Source: CAD feature listing. Evaluate the final solid. Frame: model axes, mm. Round coordinates to 2 decimals unless told otherwise and drop trailing zeros. Write each loop counter-clockwise with the first axis right and the second up, starting at its lowest first coordinate (ties: lowest second). Pieces come first, ordered by that corner, then holes. Notation, with made-up numbers: (32, 40) - (40, 40) arc R30 ccw to (40, 75) - close; hole circle Ø4 at (-6.75, 32.25). An arc over 180 degrees is marked (long way). Write item = value, one per line. Start each with the question number.
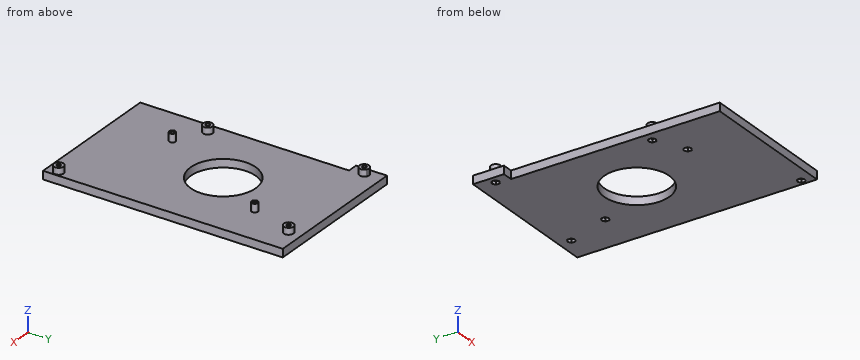
```python
from build123d import *

# Parameters (mm, degrees)
SKETCH1_R           = 20
SKETCH1_R_2         = 1.25
BOSS_EXTRUDE1_DEPTH = 5
BOSS_EXTRUDE2_START = 4
SKETCH1_3_R         = 1.25
SKETCH1_3_R_2       = 3
BOSS_EXTRUDE2_DEPTH = 4
BOSS_EXTRUDE3_START = 5
SKETCH1_5_R         = 1.9
SKETCH1_5_R_2       = 1.25
BOSS_EXTRUDE3_DEPTH = 5
CUT_EXTRUDE1_DEPTH  = 2
INTERSECT1_START    = -101.6
INTERSECT1_DEPTH    = 170


# Read off the part's stored shape, not the designer's step: Intersect1
with BuildPart() as part:
    # Sketch1 → Boss-Extrude1 (new body)
    with BuildSketch(Plane(origin=(0, 0, 0), x_dir=(0, 1, 0), z_dir=(0, 0, 1))):
        Polygon((-101.6, 25.4), (-101.6, -81.5), (215.9, -81.5), (215.9, 12.7), (196.85, 12.7), (196.85, 6.35), (-57.15, 6.35), (-57.15, 25.4), align=None)
        with Locations(Location((148.3, -36, 0), (0, 0, 270))):
            Circle(SKETCH1_R, mode=Mode.SUBTRACT)
        with Locations(Location((-92.5, 8, 0), (0, 0, 270))):
            Circle(SKETCH1_R_2, mode=Mode.SUBTRACT)
        with Locations(Location((205.3, 7.8, 0), (0, 0, 270))):
            Circle(SKETCH1_R_2, mode=Mode.SUBTRACT)
        with Locations(Location((-86.5, -73, 0), (0, 0, 270))):
            Circle(SKETCH1_R_2, mode=Mode.SUBTRACT)
        with Locations(Location((0, 0, 0), (0, 0, 270))):
            Circle(SKETCH1_R_2, mode=Mode.SUBTRACT)
        with Locations(Location((114.3, 0, 0), (0, 0, 270))):
            Circle(SKETCH1_R_2, mode=Mode.SUBTRACT)
        with Locations(Location((104.8, -18, 0), (0, 0, 270))):
            Circle(SKETCH1_R_2, mode=Mode.SUBTRACT)
        with Locations(Location((75.7, -78, 0), (0, 0, 270))):
            Circle(SKETCH1_R_2, mode=Mode.SUBTRACT)
        with Locations(Location((181.3, -56, 0), (0, 0, 270))):
            Circle(SKETCH1_R_2, mode=Mode.SUBTRACT)
        with Locations(Location((208.3, -65, 0), (0, 0, 270))):
            Circle(SKETCH1_R_2, mode=Mode.SUBTRACT)
    extrude(amount=-BOSS_EXTRUDE1_DEPTH)

    # Sketch1<3> → Boss-Extrude2 (add)
    # profile 1 of 9: a face of its own
    with BuildSketch(Plane(origin=(0, 0, 0), x_dir=(0, 1, 0), z_dir=(0, 0, 1)).offset(BOSS_EXTRUDE2_START)):
        with BuildLine():
            Line((-95.005493963, 6.35), (-89.994506037, 6.35))
            ThreePointArc((-89.994506037, 6.35), (-89.62628447, 7.13874565), (-89.5, 8))
            ThreePointArc((-89.5, 8), (-93.36125435, 10.87371553), (-95.005493963, 6.35))
        make_face()
        with Locations(Location((-92.5, 8, 0), (0, 0, 270))):
            Circle(SKETCH1_3_R, mode=Mode.SUBTRACT)
    # profile 2 of 9: a face of its own
    with BuildSketch(Plane(origin=(0, 0, 0), x_dir=(0, 1, 0), z_dir=(0, 0, 1)).offset(BOSS_EXTRUDE2_START)):
        with BuildLine():
            ThreePointArc((-95.005493963, 6.35), (-92.5, 5), (-89.994506037, 6.35))
            Line((-89.994506037, 6.35), (-95.005493963, 6.35))
        make_face()
    # profile 3 of 9: a face of its own
    with BuildSketch(Plane(origin=(0, 0, 0), x_dir=(0, 1, 0), z_dir=(0, 0, 1)).offset(BOSS_EXTRUDE2_START)):
        with Locations(Location((-86.5, -73, 0), (0, 0, 270))):
            Circle(SKETCH1_3_R_2)
        with Locations(Location((-86.5, -73, 0), (0, 0, 270))):
            Circle(SKETCH1_3_R, mode=Mode.SUBTRACT)
    # profile 4 of 9: a face of its own
    with BuildSketch(Plane(origin=(0, 0, 0), x_dir=(0, 1, 0), z_dir=(0, 0, 1)).offset(BOSS_EXTRUDE2_START)):
        with Locations(Location((0, 0, 0), (0, 0, 270))):
            Circle(SKETCH1_3_R_2)
        with Locations(Location((0, 0, 0), (0, 0, 270))):
            Circle(SKETCH1_3_R, mode=Mode.SUBTRACT)
    # profile 5 of 9: a face of its own
    with BuildSketch(Plane(origin=(0, 0, 0), x_dir=(0, 1, 0), z_dir=(0, 0, 1)).offset(BOSS_EXTRUDE2_START)):
        with Locations(Location((75.7, -78, 0), (0, 0, 270))):
            Circle(SKETCH1_3_R_2)
        with Locations(Location((75.7, -78, 0), (0, 0, 270))):
            Circle(SKETCH1_3_R, mode=Mode.SUBTRACT)
    # profile 6 of 9: a face of its own
    with BuildSketch(Plane(origin=(0, 0, 0), x_dir=(0, 1, 0), z_dir=(0, 0, 1)).offset(BOSS_EXTRUDE2_START)):
        with Locations(Location((114.3, 0, 0), (0, 0, 270))):
            Circle(SKETCH1_3_R_2)
        with Locations(Location((114.3, 0, 0), (0, 0, 270))):
            Circle(SKETCH1_3_R, mode=Mode.SUBTRACT)
    # profile 7 of 9: a face of its own
    with BuildSketch(Plane(origin=(0, 0, 0), x_dir=(0, 1, 0), z_dir=(0, 0, 1)).offset(BOSS_EXTRUDE2_START)):
        with Locations(Location((208.3, -65, 0), (0, 0, 270))):
            Circle(SKETCH1_3_R_2)
        with Locations(Location((208.3, -65, 0), (0, 0, 270))):
            Circle(SKETCH1_3_R, mode=Mode.SUBTRACT)
    # profile 8 of 9: a face of its own
    with BuildSketch(Plane(origin=(0, 0, 0), x_dir=(0, 1, 0), z_dir=(0, 0, 1)).offset(BOSS_EXTRUDE2_START)):
        with BuildLine():
            ThreePointArc((208.3, 7.8), (204.551310342, 10.705075523), (202.673690803, 6.35))
            Line((202.673690803, 6.35), (207.926309197, 6.35))
            ThreePointArc((207.926309197, 6.35), (208.205075523, 7.051310342), (208.3, 7.8))
        make_face()
        with Locations(Location((205.3, 7.8, 0), (0, 0, 270))):
            Circle(SKETCH1_3_R, mode=Mode.SUBTRACT)
    # profile 9 of 9: a face of its own
    with BuildSketch(Plane(origin=(0, 0, 0), x_dir=(0, 1, 0), z_dir=(0, 0, 1)).offset(BOSS_EXTRUDE2_START)):
        with BuildLine():
            Line((207.926309197, 6.35), (202.673690803, 6.35))
            ThreePointArc((202.673690803, 6.35), (205.3, 4.8), (207.926309197, 6.35))
        make_face()
    extrude(amount=-BOSS_EXTRUDE2_DEPTH)

    # Sketch1<5> → Boss-Extrude3 (add)
    # profile 1 of 2: a face of its own
    with BuildSketch(Plane(origin=(0, 0, 0), x_dir=(0, 1, 0), z_dir=(0, 0, 1)).offset(BOSS_EXTRUDE3_START)):
        with Locations(Location((104.8, -18, 0), (0, 0, 270))):
            Circle(SKETCH1_5_R)
        with Locations(Location((104.8, -18, 0), (0, 0, 270))):
            Circle(SKETCH1_5_R_2, mode=Mode.SUBTRACT)
    # profile 2 of 2: a face of its own
    with BuildSketch(Plane(origin=(0, 0, 0), x_dir=(0, 1, 0), z_dir=(0, 0, 1)).offset(BOSS_EXTRUDE3_START)):
        with Locations(Location((181.3, -56, 0), (0, 0, 270))):
            Circle(SKETCH1_5_R)
        with Locations(Location((181.3, -56, 0), (0, 0, 270))):
            Circle(SKETCH1_5_R_2, mode=Mode.SUBTRACT)
    extrude(amount=-BOSS_EXTRUDE3_DEPTH)

    # Sketch3 → Cut-Extrude1 (cut)
    with BuildSketch(Plane(origin=(0, 0, -5), x_dir=(1, 0, 0), z_dir=(0, 0, -1))):
        Polygon((78, -78.067136104), (80.05, -76.883568052), (80.05, -74.516431948), (78, -73.332863896), (75.95, -74.516431948), (75.95, -76.883568052), align=None)
        Polygon((65, -210.667136104), (67.05, -209.483568052), (67.05, -207.116431948), (65, -205.932863896), (62.95, -207.116431948), (62.95, -209.483568052), align=None)
        Polygon((56, -183.667136104), (58.05, -182.483568052), (58.05, -180.116431948), (56, -178.932863896), (53.95, -180.116431948), (53.95, -182.483568052), align=None)
        Polygon((-7.8, -207.667136104), (-5.75, -206.483568052), (-5.75, -204.116431948), (-7.8, -202.932863896), (-9.85, -204.116431948), (-9.85, -206.483568052), align=None)
        Polygon((0, -116.667136104), (2.05, -115.483568052), (2.05, -113.116431948), (0, -111.932863896), (-2.05, -113.116431948), (-2.05, -115.483568052), align=None)
        Polygon((18, -107.167136104), (20.05, -105.983568052), (20.05, -103.616431948), (18, -102.432863896), (15.95, -103.616431948), (15.95, -105.983568052), align=None)
        Polygon((0, -2.367136104), (2.05, -1.183568052), (2.05, 1.183568052), (0, 2.367136104), (-2.05, 1.183568052), (-2.05, -1.183568052), align=None)
        Polygon((-8, 90.132863896), (-5.95, 91.316431948), (-5.95, 93.683568052), (-8, 94.867136104), (-10.05, 93.683568052), (-10.05, 91.316431948), align=None)
        Polygon((73, 84.132863896), (75.05, 85.316431948), (75.05, 87.683568052), (73, 88.867136104), (70.95, 87.683568052), (70.95, 85.316431948), align=None)
    extrude(amount=-CUT_EXTRUDE1_DEPTH, mode=Mode.SUBTRACT)

    # Intersect1 outline → Intersect1 (cut)
    with BuildSketch(Plane(origin=(0, 0, 0), x_dir=(1, 0, 0), z_dir=(0, 1, 0)).offset(INTERSECT1_START)):
        Polygon((83, -4), (83, 6), (75.05, 6), (75.05, 5), (-10.05, 5), (-10.05, 6), (-27, 6), (-27, -4), align=None)
    extrude(amount=INTERSECT1_DEPTH, mode=Mode.SUBTRACT)


solid = part.part
```
(1) Section C-C (x = 50). Return the cut outline in (y, z).
(2) Section A-A (z = 2.5). Count the separate pieces of the cut face and the enclosed holes in it, plus the area to 3 significant figures.
(3) Ray query, L1, parallel to Y at x = 78, z = 0.5; L2, parallel to Y at x = 36, z = -1.85; L3, parallel to X at y = 181.3, z = -0.75. Return the intervals inside material, ascending. Write a range as from..to.
(4) Section B-B (y = 162.5). Return the cut outline in (x, z), plus the area to 3 significant figures.
(5) Contact query for flat-ended pins moving along their axis: P1, Ø4, axis at y = 150, z = -2, coming from the -X side; P2, Ø3, axis at x = 78, y = 75.7, coming from the -Z side; P3, Ø4.5, axis at x = -0.5, y = 113.5, coming from the -Z side; P4, Ø1.2, axis at x = -8, y = 205.5, coming from the -Z side. Output: stop coordinate, or through.
Solution:
q1.outline = (68.4, -5) - (134.02, -5) - (134.02, 0) - (68.4, 0) - close; (162.58, -5) - (215.9, -5) - (215.9, 0) - (162.58, 0) - close
q2.separate_pieces = 6
q2.enclosed_holes = 6
q2.area = 106 mm^2
q3.L1 = 72.7..74.45, 76.95..78.7
q3.L2 = 68.4..128.3, 168.3..215.9
q3.L3 = -6.35..54.75, 57.25..81.5
q4.outline = (-6.35, -5) - (21.92, -5) - (21.92, 0) - (-6.35, 0) - close; (50.08, -5) - (81.5, -5) - (81.5, 0) - (50.08, 0) - close
q4.area = 298 mm^2
q5.P1 = -6.35
q5.P2 = -3
q5.P3 = -5
q5.P4 = through
